The listing builds one solid part. Answer for the finished solid, in the listing's coordinates (mm). A direction names the side the tool comes from. Round coordinates to 2 decimals unless told otherwise and drop trailing zeros. Loops run counter-clockwise (first coordinate to the right, second up) from the corner with the lowest first, then second, coordinate; pieces in that order, holes last. Notation, with made-up numbers: (14.25, -26) - (35.25, -26) arc R15 cw to (35.25, -8) - close; hole circle Ø10 at (-37.75, -6.5). An arc over 180 degrees is marked (long way). Write item = value, one per line. Start each with the question number.
1) A tool of negligible diameter and unlimited length cuts with its end or side. For faces 1 (the flat face through (6.565, 0.5, -3.7)), 2 (the flat face through (5, 0, -5)), from which of +Z, -Z, +X, -X, +Y, -Y can it reach the whole face along a straight path? Write none if from no direction.
2) Section D-D, the plane x = 5.5 is taken. Determine the outline of the cut face in (y, z).
3) Given pin 1 Ø1.2 at (x, z) = (8, -9) entering from -Y, flat-ended and moving along its own axis, determine where the tip first touches the part or whether it passes through.
4) Straight lines are drawn through the part: line 1 along Z through (x, y) = (4, 0.45); line 2 along X through (y, z) = (0.35, -8); line 3 along X through (y, z) = (0.85, -6.25). For each, find the intervals that lie inside material, in ascending order.
5) Section A-A, the plane x = 6.75 is taken. Determine the outline of the cut face in (y, z).
6) For a pull along Z with two mould halves and no side action, classify faces 3 (the flat face through (6.308, 0.5, -5.6)), 4 (the flat face through (5, 3, -5)) as released by +Z, released by -Z, zero draft, split by the parting line, or undercut.
7) Section C-C, the plane y = 0.45 is taken. Give the number of separate pieces and of enclosed holes in the cut face, and give its area (3 significant figures).
8) Section B-B, the plane z = -4.75 is taken. Determine the outline of the cut face in (x, y).
from build123d import *

# Parameters (mm, degrees)
SKETCH_1_W          = 10
SKETCH_1_H          = 10
EXTRUDE_1_DEPTH     = 3
SKETCH_2_W          = 0.84464817
SKETCH_2_H          = 0.749284667
SKETCH_2_W_2        = 0.980881746
SKETCH_2_W_3        = 1.157985395
SKETCH_2_H_2        = 0.899141601
SKETCH_2_W_4        = 1.771036487
SKETCH_2_H_3        = 1.062621892
SKETCH_2_W_5        = 1.253348898
SKETCH_2_H_4        = 1.675672983
SKETCH_2_W_6        = 0.408700727
SKETCH_2_H_5        = 2.070750353
SKETCH_2_W_7        = 1.416829189
SKETCH_2_H_6        = 1.171608752
SKETCH_2_W_8        = 1.593932837
SKETCH_2_H_7        = 1.212478826
CUT_EXTRUDE_1_DEPTH = 1
SKETCH_3_W          = 0.351704959
SKETCH_3_H          = 0.859723233
SKETCH_3_W_2        = 0.371244123
SKETCH_3_H_2        = 1.543593986
SKETCH_3_W_3        = 1.445898165
SKETCH_3_H_3        = 0.429861616
SKETCH_3_W_4        = 1.016036548
SKETCH_3_H_4        = 1.055114877
SKETCH_3_W_5        = 1.11373237
SKETCH_3_H_5        = 0.840184069
SKETCH_3_H_6        = 0.937879891
CUT_EXTRUDE_3_DEPTH = 1


with BuildPart() as part:
    # 草图1 → 凸台-拉伸1 (new body)
    with BuildSketch(Plane(origin=(0, 0, 0), x_dir=(1, 0, 0), z_dir=(0, 1, 0))):
        with Locations((5, 5)):
            Rectangle(SKETCH_1_W, SKETCH_1_H)
    extrude(amount=EXTRUDE_1_DEPTH)

    # 草图2 → 切除-拉伸1 (cut)
    with BuildSketch(Plane(origin=(0, 0, 0), x_dir=(1, 0, 0), z_dir=(0, 1, 0))):
        with Locations((1.130966445, 8.841786839)):
            Rectangle(SKETCH_2_W, SKETCH_2_H)
        with Locations((4.713909491, 8.841786839)):
            Rectangle(SKETCH_2_W_2, SKETCH_2_H)
        with Locations((1.451115349, 0.851687615)):
            Rectangle(SKETCH_2_W_3, SKETCH_2_H_2)
        with Locations((8.419462755, 8.685118227)):
            Rectangle(SKETCH_2_W_4, SKETCH_2_H_3)
        with Locations((3.923754751, 6.362335759)):
            Rectangle(SKETCH_2_W_5, SKETCH_2_H_4)
        with Locations((6.103491964, 5.647109485)):
            Rectangle(SKETCH_2_W_6, SKETCH_2_H_5)
        with Locations((4.005494897, 3.712592708)):
            Rectangle(SKETCH_2_W_7, SKETCH_2_H_6)
        with Locations((5.51087591, 2.261705125)):
            Rectangle(SKETCH_2_W_8, SKETCH_2_H_7)
    extrude(amount=CUT_EXTRUDE_1_DEPTH, mode=Mode.SUBTRACT)

    # 草图3 → 切除-拉伸3 (cut)
    with BuildSketch(Plane(origin=(0, 0, 0), x_dir=(1, 0, 0), z_dir=(0, 1, 0))):
        with Locations((1.934516979, 4.887785167)):
            Rectangle(SKETCH_3_W, SKETCH_3_H)
        with Locations((2.29599152, 7.39856779)):
            Rectangle(SKETCH_3_W_2, SKETCH_3_H_2)
        with Locations((4.415990856, 7.955433975)):
            Rectangle(SKETCH_3_W_3, SKETCH_3_H_3)
        with Locations((7.483639664, 6.099213359)):
            Rectangle(SKETCH_3_W_4, SKETCH_3_H_4)
        with Locations((7.122165123, 3.686126557)):
            Rectangle(SKETCH_3_W_5, SKETCH_3_H_5)
        with Locations((7.815805458, 2.210919646)):
            Rectangle(SKETCH_3_W_4, SKETCH_3_H_6)
    extrude(amount=CUT_EXTRUDE_3_DEPTH, mode=Mode.SUBTRACT)


solid = part.part
Geometry check:
q1.face_1 = -Y
q1.face_2 = +Z, -Z, +X, -X, -Y
q2.outline = (0, -10) - (3, -10) - (3, 0) - (0, 0) - (0, -1.66) - (1, -1.66) - (1, -2.87) - (0, -2.87) - close
q3.pin_1 = 0
q4.line_1 = -10 to -8.17, -7.74 to -7.2, -5.52 to -4.3, -3.13 to 0
q4.line_2 = 0 to 2.11, 2.48 to 3.69, 5.14 to 10
q4.line_3 = 0 to 3.3, 4.55 to 5.9, 6.31 to 6.98, 7.99 to 10
q5.outline = (0, -10) - (3, -10) - (3, 0) - (0, 0) - (0, -3.27) - (1, -3.27) - (1, -4.11) - (0, -4.11) - close
q6.face_3 = undercut
q6.face_4 = zero draft
q7.separate_pieces = 1
q7.enclosed_holes = 14
q7.area = 84.7 mm2
q8.outline = (0, 0) - (1.76, 0) - (1.76, 1) - (2.11, 1) - (2.11, 0) - (5.9, 0) - (5.9, 1) - (6.31, 1) - (6.31, 0) - (10, 0) - (10, 3) - (0, 3) - close
